Can you work these out from the model? Positions are in its coordinate system, mm. Face numbers are marked on the shaded views. A direction names the side the tool comes from. Give positions to 0.01 mm unless a question says otherwise; leave off trailing zeros. Order: outer loops, then holes, each group sorted by start corner. A loop starts at its lowest first (then second) coordinate and runs counter-clockwise, first axis right, second up. Notation, with made-up numbers: (-15, 75) - (-11, 75) arc R15 ccw to (-11, 87) - close; hole circle Ø7 at (35, 76.5). An arc over 180 degrees is marked (long way). Use one line per item in the form item = value. Start each with the question number.
1) For pin 1 (4 mm diameter, centred on x = -14.94, z = -3.5, fed in from +Y); pin 2 (5 mm diameter, centred on x = -37.5, z = -1.5, fed in from -Y); pin 3 (5 mm diameter, centred on x = -5.5, z = -4.5, fed in from +Y); pin 4 (10 mm diameter, centred on x = -38, y = 24.5, fed in from +Z), each with a flat end and sliding along its axis, tell me the tip position at first contact or that it passes through.
2) Suppose I cut it at A-A, the plane z = -3.5. Write out the boundary of the cut face in (x, y), and give its area (3 significant figures).
3) Please list where these lines run through material, in increasing order: probe 1 along X at (y, z) = (-5.5, -3.5); probe 2 along Z at (x, y) = (-15.5, 17); probe 3 along Y at (x, z) = (-34, 2).
4) Which directions (+Z, -Z, +X, -X, +Y, -Y) give clear straight access to the entire face, cutting with the end or side of a thin tool? Please do the marked faces 1 and 2.
5) Suppose I cut it at D-D, the plane y = -1.5. Write out the boundary of the cut face in (x, z).
6) Suppose I cut it at B-B, the plane x = -39. Write out the boundary of the cut face in (y, z), and give its area (3 significant figures).
7) Suppose I cut it at C-C, the plane z = 2. Write out the boundary of the cut face in (x, y), and give its area (3 significant figures).
```python
from build123d import *

# Parameters (mm, degrees)
CROQUIS1_R              = 8.05
SALIENTE_EXTRUIR1_DEPTH = 3
CROQUIS2_W              = 20
CROQUIS2_H              = 3
SALIENTE_EXTRUIR2_DEPTH = 11
CROQUIS3_R              = 1.5
CORTAR_EXTRUIR1_DEPTH   = 3
REDONDEO2_R             = 2
CROQUIS4_R              = 2.25
CORTAR_EXTRUIR2_DEPTH   = 1


with BuildPart() as part:
    # Croquis1 → Saliente-Extruir1 (new body)
    with BuildSketch(Plane.XY):
        with BuildLine():
            Line((-30.938838255, -8.045633461), (-10.938838255, -8.045633461))
            Line((-10.938838255, -8.045633461), (-10.938838255, -7.045633461))
            ThreePointArc((-10.938838255, -7.045633461), (-10.353051818, -5.631419899), (-8.938838255, -5.045633461))
            Line((-8.938838255, -5.045633461), (9.549778797, -5.045633461))
            ThreePointArc((9.549778797, -5.045633461), (10.972041616, -4.456512912), (11.561162165, -3.034250093))
            Line((11.561162165, -3.034250093), (11.561162165, 39.954366539))
            ThreePointArc((11.561162165, 39.954366539), (10.968432365, 41.078847271), (9.963268776, 41.856942185))
            ThreePointArc((9.963268776, 41.856942185), (2.408997489, 45.151653306), (-0.316073105, 52.929578886))
            ThreePointArc((-0.316073105, 52.929578886), (-9.509697497, 51.145023059), (-17.59663302, 46.421799285))
            ThreePointArc((-17.59663302, 46.421799285), (-21.556040731, 49.695374216), (-23.633455433, 54.394049605))
            ThreePointArc((-23.633455433, 54.394049605), (-28.98150225, 52.459242343), (-33.559009638, 49.084111234))
            ThreePointArc((-33.559009638, 49.084111234), (-34.606059472, 51.579310047), (-33.582063508, 54.084058086))
            ThreePointArc((-33.582063508, 54.084058086), (-40.220863613, 51.667488325), (-45.549660534, 47.028803207))
            ThreePointArc((-45.549660534, 47.028803207), (-46.044361143, 49.705869681), (-45.402636247, 52.35154592))
            ThreePointArc((-45.402636247, 52.35154592), (-50.909137078, 48.962948767), (-53.438838255, 43.012759358))
            Line((-53.438838255, 43.012759358), (-53.438838255, -2.988324387))
            ThreePointArc((-53.438838255, -2.988324387), (-52.861811755, -4.429826639), (-51.430168576, -5.030897458))
            Line((-51.430168576, -5.030897458), (-32.937399988, -5.044196229))
            ThreePointArc((-32.937399988, -5.044196229), (-31.52411628, -5.630490745), (-30.938838255, -7.044195711))
            Line((-30.938838255, -7.044195711), (-30.938838255, -8.045633461))
        make_face()
        with Locations((-7.938838255, 24.954366539)):
            Circle(CROQUIS1_R, mode=Mode.SUBTRACT)
        with Locations((-33.938838255, 24.954366539)):
            Circle(CROQUIS1_R, mode=Mode.SUBTRACT)
    extrude(amount=SALIENTE_EXTRUIR1_DEPTH)

    # Croquis2 → Saliente-Extruir2 (add)
    with BuildSketch(Plane.XY.offset(3)):
        with Locations((-20.938838255, -6.545633461)):
            Rectangle(CROQUIS2_W, CROQUIS2_H)
    extrude(amount=-SALIENTE_EXTRUIR2_DEPTH)

    # Croquis3 → Cortar-Extruir1 (cut)
    with BuildSketch(Plane(origin=(0, -5.045633461, 0), x_dir=(1, 0, 0), z_dir=(0, 1, 0))):
        with Locations((-14.938838255, 3.5)):
            Circle(CROQUIS3_R)
        with Locations((-26.938838255, 3.5)):
            Circle(CROQUIS3_R)
    extrude(amount=-CORTAR_EXTRUIR1_DEPTH, mode=Mode.SUBTRACT)

    # Redondeo2
    redondeo2_edges = [part.edges().sort_by_distance(p)[0] for p in [
        (-30.938838255, -6.545633461, -8),
        (-10.938838255, -6.545633461, -8),
    ]]
    fillet(redondeo2_edges, radius=REDONDEO2_R)

    # Croquis4 → Cortar-Extruir2 (cut)
    with BuildSketch(Plane(origin=(0, -5.045633461, 0), x_dir=(1, 0, 0), z_dir=(0, 1, 0))):
        with Locations((-26.938838255, 3.5)):
            Circle(CROQUIS4_R)
        with Locations((-14.938838255, 3.5)):
            Circle(CROQUIS4_R)
    extrude(amount=-CORTAR_EXTRUIR2_DEPTH, mode=Mode.SUBTRACT)


solid = part.part
```
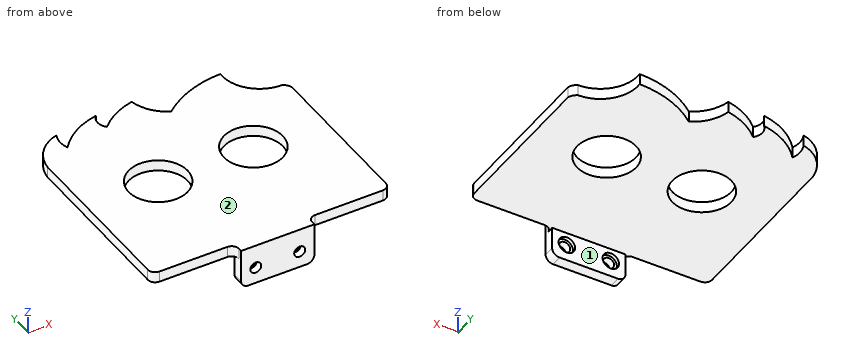
Result sheet:
q1.pin_1 = -6.05
q1.pin_2 = -5.04
q1.pin_3 = through
q1.pin_4 = 3
q2.outline = (-30.94, -8.05) - (-28.44, -8.05) - (-28.44, -6.05) - (-29.19, -6.05) - (-29.19, -5.05) - (-30.94, -5.05) - close; (-25.44, -8.05) - (-16.44, -8.05) - (-16.44, -6.05) - (-17.19, -6.05) - (-17.19, -5.05) - (-24.69, -5.05) - (-24.69, -6.05) - (-25.44, -6.05) - close; (-13.44, -8.05) - (-10.94, -8.05) - (-10.94, -5.05) - (-12.69, -5.05) - (-12.69, -6.05) - (-13.44, -6.05) - close
q2.area = 39.0 mm²
q3.probe_1 = -30.94 to -29.19, -24.69 to -17.19, -12.69 to -10.94
q3.probe_2 = 0 to 3
q3.probe_3 = -5.04 to 16.9, 33 to 49.62, 53.58 to 54.01
q4.face_1 = -Z, +X, -X, +Y
q4.face_2 = +Z, +X, -X, +Y, -Y
q5.outline = (-53.44, 0) - (11.56, 0) - (11.56, 3) - (-53.44, 3) - close
q6.outline = (-5.04, 0) - (18.69, 0) - (18.69, 3) - (-5.04, 3) - close; (31.21, 0) - (52.33, 0) - (52.33, 3) - (31.21, 3) - close
q6.area = 135 mm²
q7.outline = (-53.44, -2.99) arc R2.01 ccw to (-51.43, -5.03) - (-32.94, -5.04) arc R2 cw to (-30.94, -7.04) - (-30.94, -8.05) - (-10.94, -8.05) - (-10.94, -7.05) arc R2 cw to (-8.94, -5.05) - (9.55, -5.05) arc R2.01 ccw to (11.56, -3.03) - (11.56, 39.95) arc R3 ccw to (9.96, 41.86) arc R10.31 cw to (-0.32, 52.93) arc R27.93 ccw to (-17.6, 46.42) arc R11.18 cw to (-23.63, 54.39) arc R19.8 ccw to (-33.56, 49.08) arc R3.54 cw to (-33.58, 54.08) arc R19.35 ccw to (-45.55, 47.03) arc R6.52 cw to (-45.4, 52.35) arc R10.64 ccw to (-53.44, 43.01) - close; hole circle Ø16.1 at (-33.94, 24.95); hole circle Ø16.1 at (-7.94, 24.95)
q7.area = 3,200 mm²
